Part model, mm, in its own coordinate system. Face numbers are marked on the shaded views. Coordinates: 2 decimals unless noted, no trailing zeros. Loops run counter-clockwise (first coordinate to the right, second up) from the corner with the lowest first, then second, coordinate; pieces in that order, holes last. Notation, with made-up numbers: (70, 68) - (92, 68) arc R17 ccw to (92, 85) - close; hole circle Ø11 at (61.25, 31). An arc over 180 degrees is marked (long way). Use a Markdown table: item, result. Add a question column.
1) Pull direction X, two halves, no side cores. Call the marked faces 1, 2, 3 and 4: +X half, -X half, draft (parallel to the pull), parting line (faces both ways), or undercut.
2) Drop a flat-ended pin along its axis: P1, Ø12, axis at x = -18.5, y = -15, coming from the -Z side. Give the stop position or say it passes through.
3) Band-saw the part on B-B (y = 0). Give the cut face in (x, z), plus the area to 3 significant figures.
4) Band-saw the part on A-A (x = 0). Give the cut face in (y, z), plus the area to 3 significant figures.
5) Probe probe 1 along Y at (x, z) = (0, 19.75); probe 2 along Y at (x, z) = (-8, 13); probe 3 along X at (y, z) = (-12, 9.75). List the from-to ranges inside material, lowest first. Write a range as [from, to].
6) Band-saw the part on C-C (z = 4). Give the cut face in (x, y).
Autodesk Inventor part; units mm, degrees
ref_plane "YZ Plane" through (0, 0, 0) normal (1, 0, 0) x (0, 1, 0)
ref_plane "XZ Plane" through (0, 0, 0) normal (0, 1, 0) x (-1, 0, 0)
ref_plane "XY Plane" through (0, 0, 0) normal (0, 0, 1) x (1, 0, 0)
sketch "Sketch1" plane through (0, 0, 0) normal (0, 0, 1) x (1, 0, 0)
  line L0 (-50, 75) -> (50, 75)
  line L1 (50, 75) -> (50, -75)
  line L2 (50, -75) -> (-50, -75)
  line L3 (-50, -75) -> (-50, 75)
  point P0 (0, 0)
  point P1 (0, 75)
  point P2 (-50, 0)
  dimension "d0" = 100
  dimension "d1" = 150
extrude "Extrusion1" add sketch "Sketch1" along normal blind 25
sketch "Sketch2" plane through (0, 0, 25) normal (0, 0, 1) x (1, 0, 0)
  line L0 (50, 75) -> (-50, 75)
  line L1 (-50, -75) -> (50, -75)
  line L2 (-50, 75) -> (50, -75) construction
  circle A0 centre (0, 0) radius 19
  dimension "d4" = 38
extrude "Extrusion2" cut sketch "Sketch2" against normal through all
properties part number "Foam_Top_Big_Mic" material "Polystyrene, Expanded"
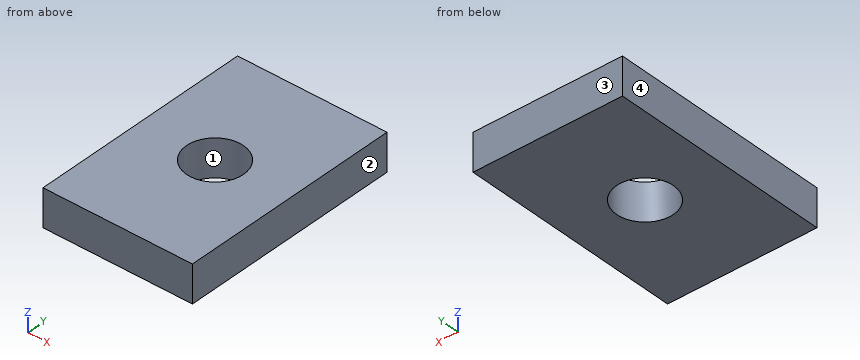
Answer block:
| question | item | result |
|---|---|---|
| 1 | face 1 | undercut |
| 1 | face 2 | +X half |
| 1 | face 3 | draft |
| 1 | face 4 | -X half |
| 2 | P1 | z = 0 |
| 3 | outline | (-50, 0) - (-19, 0) - (-19, 25) - (-50, 25) - close; (19, 0) - (50, 0) - (50, 25) - (19, 25) - close |
| 3 | area | 1,550 mm2 |
| 4 | outline | (-75, 0) - (-19, 0) - (-19, 25) - (-75, 25) - close; (19, 0) - (75, 0) - (75, 25) - (19, 25) - close |
| 4 | area | 2,800 mm2 |
| 5 | probe 1 | [-75, -19], [19, 75] |
| 5 | probe 2 | [-75, -17.23], [17.23, 75] |
| 5 | probe 3 | [-50, -14.73], [14.73, 50] |
| 6 | outline | (-50, -75) - (50, -75) - (50, 75) - (-50, 75) - close; hole circle Ø38 at (0, 0) |
